```python
from build123d import *

# Parameters (mm, degrees)
SKETCH1_W           = 40
SKETCH1_H           = 40
BOSS_EXTRUDE1_DEPTH = 11
FILLET1_R           = 4
FILLET2_R           = 4
FILLET3_R           = 4
FILLET4_R           = 4
SKETCH2_R           = 19
CUT_EXTRUDE1_DEPTH  = 11
CUT_EXTRUDE2_DEPTH  = 8
SKETCH4_R           = 1.5
CUT_EXTRUDE3_DEPTH  = 11


with BuildPart() as part:
    # Sketch1 → Boss-Extrude1 (new body)
    with BuildSketch(Plane(origin=(0, 0, 0), x_dir=(1, 0, 0), z_dir=(0, 1, 0))):
        with Locations((20, 20)):
            Rectangle(SKETCH1_W, SKETCH1_H)
    extrude(amount=BOSS_EXTRUDE1_DEPTH)

    # Fillet1
    fillet1_edges = [part.edges().sort_by_distance(p)[0] for p in [
        (40, 5.5, 0),
    ]]
    fillet(fillet1_edges, radius=FILLET1_R)

    # Fillet2
    fillet2_edges = [part.edges().sort_by_distance(p)[0] for p in [
        (0, 5.5, 0),
    ]]
    fillet(fillet2_edges, radius=FILLET2_R)

    # Fillet3
    fillet3_edges = [part.edges().sort_by_distance(p)[0] for p in [
        (0, 5.5, -40),
    ]]
    fillet(fillet3_edges, radius=FILLET3_R)

    # Fillet4
    fillet4_edges = [part.edges().sort_by_distance(p)[0] for p in [
        (40, 5.5, -40),
    ]]
    fillet(fillet4_edges, radius=FILLET4_R)

    # Sketch2 → Cut-Extrude1 (cut)
    with BuildSketch(Plane(origin=(0, 11, 0), x_dir=(1, 0, 0), z_dir=(0, 1, 0))):
        with Locations(Location((20, 20, 0), (0, 0, 270))):
            Circle(SKETCH2_R)
    extrude(amount=-CUT_EXTRUDE1_DEPTH, mode=Mode.SUBTRACT)

    # Sketch3 → Cut-Extrude2 (cut)
    with BuildSketch(Plane(origin=(0, 11, 0), x_dir=(1, 0, 0), z_dir=(0, 1, 0))):
        with BuildLine():
            Line((4, 32), (0, 36))
            Line((0, 36), (0, 20))
            ThreePointArc((0, 20), (1.026334039, 26.32455532), (4, 32))
        make_face()
        with BuildLine():
            Line((4, 40), (8, 36))
            ThreePointArc((8, 36), (13.67544468, 38.973665961), (20, 40))
            Line((20, 40), (4, 40))
        make_face()
        with BuildLine():
            Line((36, 40), (20, 40))
            ThreePointArc((20, 40), (26.32455532, 38.973665961), (32, 36))
            Line((32, 36), (36, 40))
        make_face()
        with BuildLine():
            Line((40, 36), (36, 32))
            ThreePointArc((36, 32), (38.973665961, 26.32455532), (40, 20))
            Line((40, 20), (40, 36))
        make_face()
        with BuildLine():
            Line((40, 4), (40, 20))
            ThreePointArc((40, 20), (38.973665961, 13.67544468), (36, 8))
            Line((36, 8), (40, 4))
        make_face()
        with BuildLine():
            ThreePointArc((32, 4), (26.32455532, 1.026334039), (20, 0))
            Line((20, 0), (36, 0))
            Line((36, 0), (32, 4))
        make_face()
        with BuildLine():
            ThreePointArc((20, 0), (13.67544468, 1.026334039), (8, 4))
            Line((8, 4), (4, 0))
            Line((4, 0), (20, 0))
        make_face()
        with BuildLine():
            ThreePointArc((4, 8), (1.026334039, 13.67544468), (0, 20))
            Line((0, 20), (0, 4))
            Line((0, 4), (4, 8))
        make_face()
    extrude(amount=-CUT_EXTRUDE2_DEPTH, mode=Mode.SUBTRACT)

    # Sketch4 → Cut-Extrude3 (cut)
    with BuildSketch(Plane(origin=(0, 11, 0), x_dir=(1, 0, 0), z_dir=(0, 1, 0))):
        with Locations(Location((36, 36, 0), (0, 0, 270))):
            Circle(SKETCH4_R)
        with Locations(Location((4, 36, 0), (0, 0, 270))):
            Circle(SKETCH4_R)
        with Locations(Location((4, 4, 0), (0, 0, 270))):
            Circle(SKETCH4_R)
        with Locations(Location((36, 4, 0), (0, 0, 270))):
            Circle(SKETCH4_R)
    extrude(amount=-CUT_EXTRUDE3_DEPTH, mode=Mode.SUBTRACT)


solid = part.part
```
Geometry check sheet. Reference: the model listing, model coordinates, mm. A direction names the side the tool comes from. Coordinates: 2 decimals unless noted, no trailing zeros. Order: outer loops, then holes, each group sorted by start corner. A loop starts at its lowest first (then second) coordinate and runs counter-clockwise, first axis right, second up. Notation, with made-up numbers: M 43,-6.5 L 98,-6.5 A19 ccw 98,16.5 Z; hole C 54.5,-0.75 d10. An arc over 180 degrees is marked long. One line per question, with ' | ' between items. Start each with the question number.
Item 1: Cross-section at D-D on y = 7. Enter the section's corners in (x, z), then the cut area to 3 significant figures.
Item 2: Cross-section at B-B on x = 10.5. Enter the section's corners in (y, z).
Item 3: Material ranges on L1, parallel to X at y = 4.75, z = -36.5; L2, parallel to X at y = 2.75, z = -4; L3, parallel to X at y = 4.5, z = -34, recorded low to high. Write a range as [from, to].
Item 4: Cross-section at A-A on y = 2.5. Enter the section's corners in (x, z), then the cut area to 3 significant figures.
Item 5: Set-up check for faces 1 (the cylindrical face through (34.536, 5.577, -4.325)), 2 (the flat face through (30, 3, -39)), 3 (the flat face through (39, 3, -10)), 4 (the flat face through (40, 1, -20)), 5 (the flat face through (1, 3, -32)): record each of +Z, -Z, +X, -X, +Y, -Y from which the full face is reachable in a straight line by a thin tool's end or side.
Item 6: Gauge pin test, flat end, axial feed: pin 1 (4 mm diameter, centred on y = 7.5, z = -9.5, fed in from -X). Record the tip position at first contact, or that the pin passes through.
Item 7: Cross-section at C-C on z = -34. Enter the section's corners in (x, y), then the cut area to 3 significant figures.
Item 8: Draft check along X on faces 6 (the flat face through (38, 7, -6)), 7 (the flat face through (8, 0, -35)), 8 (the flat face through (8, 3, -39)), 9 (the flat face through (6, 7, -38)). Enter one of: pulls with the +X half, pulls with the -X half, needs draft (parallel to the pull), parting line crosses it, or undercut.
Findings:
1) outline: M 0,-36 A4 ccw 4,-40 L 8,-36 A20 ccw 32,-36 L 36,-40 A4 ccw 40,-36 L 36,-32 A20 ccw 36,-8 L 40,-4 A4 ccw 36,0 L 32,-4 A20 ccw 8,-4 L 4,0 A4 ccw 0,-4 L 4,-8 A20 ccw 4,-32 Z; hole C 20,-20 d38; hole C 4,-36 d3; hole C 4,-4 d3; hole C 36,-36 d3; hole C 36,-4 d3 | area: 237 mm²
2) outline: M 0,-40 L 3,-40 L 3,-37.6 L 11,-37.6 L 11,-36.45 L 0,-36.45 Z; M 0,-3.55 L 11,-3.55 L 11,-2.4 L 3,-2.4 L 3,0 L 0,0 Z
3) L1: x = [0.03, 2.59], [5.41, 7.5], [8.7, 10.58], [29.42, 31.3], [32.5, 34.59], [37.41, 39.97] | L2: x = [0, 2.5], [5.5, 9.75], [30.25, 34.5], [37.5, 40] | L3: x = [2, 7.15], [32.85, 38]
4) outline: M 0,-36 A4 ccw 4,-40 L 36,-40 A4 ccw 40,-36 L 40,-4 A4 ccw 36,0 L 4,0 A4 ccw 0,-4 Z; hole C 20,-20 d38; hole C 4,-36 d3; hole C 4,-4 d3; hole C 36,-36 d3; hole C 36,-4 d3 | area: 424 mm²
5) face 1: +Y, -Y | face 2: -Z, +Y | face 3: +X, +Y | face 4: +Z, -Z, +X, +Y, -Y | face 5: -X, +Y
6) pin 1: stops at x = 1.9
7) outline: M 0,0 L 7.15,0 L 7.15,11 L 2,11 L 2,3 L 0,3 Z; M 32.85,0 L 40,0 L 40,3 L 38,3 L 38,11 L 32.85,11 Z | area: 125 mm²
8) face 6: pulls with the +X half | face 7: needs draft | face 8: undercut | face 9: undercut
